The model under review builds one solid part; all positions refer to its coordinate system, in mm. A direction names the side the tool comes from. Give positions to 0.01 mm unless a question says otherwise; leave off trailing zeros. Write each loop counter-clockwise with the first axis right and the second up, starting at its lowest first coordinate (ties: lowest second). Pieces come first, ordered by that corner, then holes. Notation, with made-up numbers: M 21.25,24 L 53.25,24 A38 ccw 53.25,63 Z; hole C -24,-6 d7. An arc over 180 degrees is marked long. Write item = value, one per line. Start each with the question number.
```python
from build123d import *

# Parameters (mm, degrees)
SKETCH_R        = 1.5
PAD_DEPTH       = 22.5
SKETCH001_R     = 1.5
POCKET_DEPTH    = 18.429932
SKETCH004_R     = 1.5
POCKET001_DEPTH = 20.136
SKETCH005_R     = 1.5
POCKET002_DEPTH = 20.136


with BuildPart() as part:
    # Sketch → Pad (new body)
    with BuildSketch(Plane.XY):
        with BuildLine():
            ThreePointArc((22.5, 0), (0, 22.5), (-22.5, 0))
            Line((-22.5, -30), (-22.5, 0))
            Line((-2.365, -30), (-22.5, -30))
            Line((-2.365, -30), (-2.365, -15))
            Line((-2.365, -15), (2.365, -15))
            Line((2.365, -15), (2.365, -30))
            Line((22.5, -30), (2.365, -30))
            Line((22.5, 0), (22.5, -30))
        make_face()
        with Locations((-10.606602, 10.606602)):
            Circle(SKETCH_R, mode=Mode.SUBTRACT)
        with Locations((-10.606602, -10.606602)):
            Circle(SKETCH_R, mode=Mode.SUBTRACT)
        with Locations((10.606602, -10.606602)):
            Circle(SKETCH_R, mode=Mode.SUBTRACT)
        with Locations((10.606602, 10.606602)):
            Circle(SKETCH_R, mode=Mode.SUBTRACT)
        with BuildLine():
            ThreePointArc((-2.5, 7.071068), (0, -7.5), (2.5, 7.071068))
            Line((2.5, 7.071068), (2.5, 4.071068))
            Line((2.5, 4.071068), (-2.5, 4.071068))
            Line((-2.5, 4.071068), (-2.5, 7.071068))
        make_face(mode=Mode.SUBTRACT)
    extrude(amount=PAD_DEPTH)

    # Sketch001 → Pocket (cut, through all)
    with BuildSketch(Plane.XZ.offset(-4.071068)):
        with Locations((0, 11.25)):
            Circle(SKETCH001_R)
    extrude(amount=-POCKET_DEPTH, mode=Mode.SUBTRACT)

    # Sketch004 → Pocket001 (cut, through all)
    with BuildSketch(Plane.YZ.offset(-2.365)):
        with Locations((-26.25, 16.875)):
            Circle(SKETCH004_R)
        with Locations((-18.75, 16.875)):
            Circle(SKETCH004_R)
        with Locations((-18.75, 5.625)):
            Circle(SKETCH004_R)
        with Locations((-26.25, 5.625)):
            Circle(SKETCH004_R)
    extrude(amount=-POCKET001_DEPTH, mode=Mode.SUBTRACT)

    # Sketch005 → Pocket002 (cut, through all)
    with BuildSketch(Plane(origin=(2.365, 0, 0), x_dir=(0, -1, 0), z_dir=(-1, 0, 0))):
        with Locations((18.694969, 16.847485)):
            Circle(SKETCH005_R)
        with Locations((26.194969, 16.847485)):
            Circle(SKETCH005_R)
        with Locations((18.694969, 5.597485)):
            Circle(SKETCH005_R)
        with Locations((26.194969, 5.597485)):
            Circle(SKETCH005_R)
    extrude(amount=-POCKET002_DEPTH, mode=Mode.SUBTRACT)


solid = part.part
```
Item 1: We need section B-B, the plane x = 0. Write out the cut boundary in (y, z), and give its area (3 significant figures).
Item 2: We need section D-D, the plane x = 13.5. Write out the cut boundary in (y, z).
Item 3: Clearance check with flat-ended pins moving along their axes: P1, Ø2, axis at x = 2, y = -13.5, coming from the -Z side; P2, Ø2.5, axis at y = 5.5, z = 8, coming from the -X side; P3, Ø10, axis at x = -14.5, z = 8, coming from the +Y side; P4, Ø1.8, axis at y = -26.25, z = 16.875, coming from the -X side. State where each tip first meets the part, or that it passes through.
Item 4: To check wall thickness, follow probe 1 along X at (y, z) = (-25, 2.25) (3 decimals); probe 2 along X at (y, z) = (6.5, 5); probe 3 along Z at (x, y) = (-13, -27). State the ranges of each line that lie inside material, in increasing order. Write a range as [from, to].
Item 5: The part is to be moulded in two halves that separate along Z. For faces 6 (the flat face through (-2, 4.071, 11)), 7 (the flat face through (0, -9, 0)), 8 (the cylindrical face through (-12.29, -20.25, 16.94)), say which applies: released by +Z, released by -Z, zero draft, split by the parting line, or undercut.
Item 6: For faces 1 (the cylindrical face through (-12.29, -20.25, 5.69)), 2 (the flat face through (2.5, 6, 11)), 3 (the flat face through (2.365, -22, 11)), 4 (the flat face through (-22.5, -15, 11)), 5 (the cylindrical face through (12.292, -27.626, 6.048)), list the 3-axis set-ups (+Z, -Z, +X, -X, +Y, -Y) from which the entire face can be reached by the end or side of a thin tool; tool diameter is ignored.
Item 7: We need section C-C, the plane z = 21.25. Write out the cut boundary in (x, y) (3 decimals).
Item 8: We need section A-A, the plane y = -16. Write out the cut boundary in (x, z) (3 decimals), and give its area (3 significant figures).
Worked out:
q1.outline = M -15,0 L -7.5,0 L -7.5,22.5 L -15,22.5 Z; M 4.07,0 L 22.5,0 L 22.5,9.75 L 4.07,9.75 Z; M 4.07,12.75 L 22.5,12.75 L 22.5,22.5 L 4.07,22.5 Z
q1.area = 528 mm²
q2.outline = M -30,0 L 18,0 L 18,22.5 L -30,22.5 Z; hole C -26.19,5.6 d3; hole C -26.19,16.85 d3; hole C -18.69,5.6 d3; hole C -18.69,16.85 d3
q3.P1 = 0
q3.P2 = -22.09
q3.P3 = 20.4
q3.P4 = through
q4.probe_1 = [-22.5, -2.365], [2.365, 22.5]
q4.probe_2 = [-21.54, -3.74], [-2.5, 2.5], [3.74, 21.54]
q4.probe_3 = [0, 4.33], [6.92, 15.58], [18.17, 22.5]
q5.face_6 = zero draft
q5.face_7 = released by -Z
q5.face_8 = undercut
q6.face_1 = -X
q6.face_2 = +Z, -Z
q6.face_3 = +Z, -Z, -Y
q6.face_4 = +Z, -Z, -X, +Y, -Y
q6.face_5 = +X
q7.outline = M -22.5,-30 L -2.365,-30 L -2.365,-15 L 2.365,-15 L 2.365,-30 L 22.5,-30 L 22.5,0 A22.5 ccw -22.5,0 Z; hole C -10.607,-10.607 d3; hole C -10.607,10.607 d3; hole M -2.5,4.071 L -2.5,7.071 A7.5 ccw long 2.5,7.071 L 2.5,4.071 Z; hole C 10.607,-10.607 d3; hole C 10.607,10.607 d3
q8.outline = M -22.5,0 L -2.365,0 L -2.365,22.5 L -22.5,22.5 Z; M 2.365,0 L 22.5,0 L 22.5,22.5 L 2.365,22.5 Z
q8.area = 906 mm²
